Here's the drawing with two shaded views (mm, measured from the low corner). I have some questions. A direction names the side the tool comes from. Round coordinates to 2 decimals unless told otherwise and drop trailing zeros. Write each loop counter-clockwise with the first axis right and the second up, starting at its lowest first coordinate (ties: lowest second). Pieces come first, ordered by that corner, then holes. Notation, with made-up numbers: (13, 55.25) - (52, 55.25) arc R28 ccw to (52, 91.25) - close; hole circle Ø2 at (49.5, 79.5). An arc over 180 degrees is marked (long way). Return JSON: item names as keys, results as strings. Group by question number.
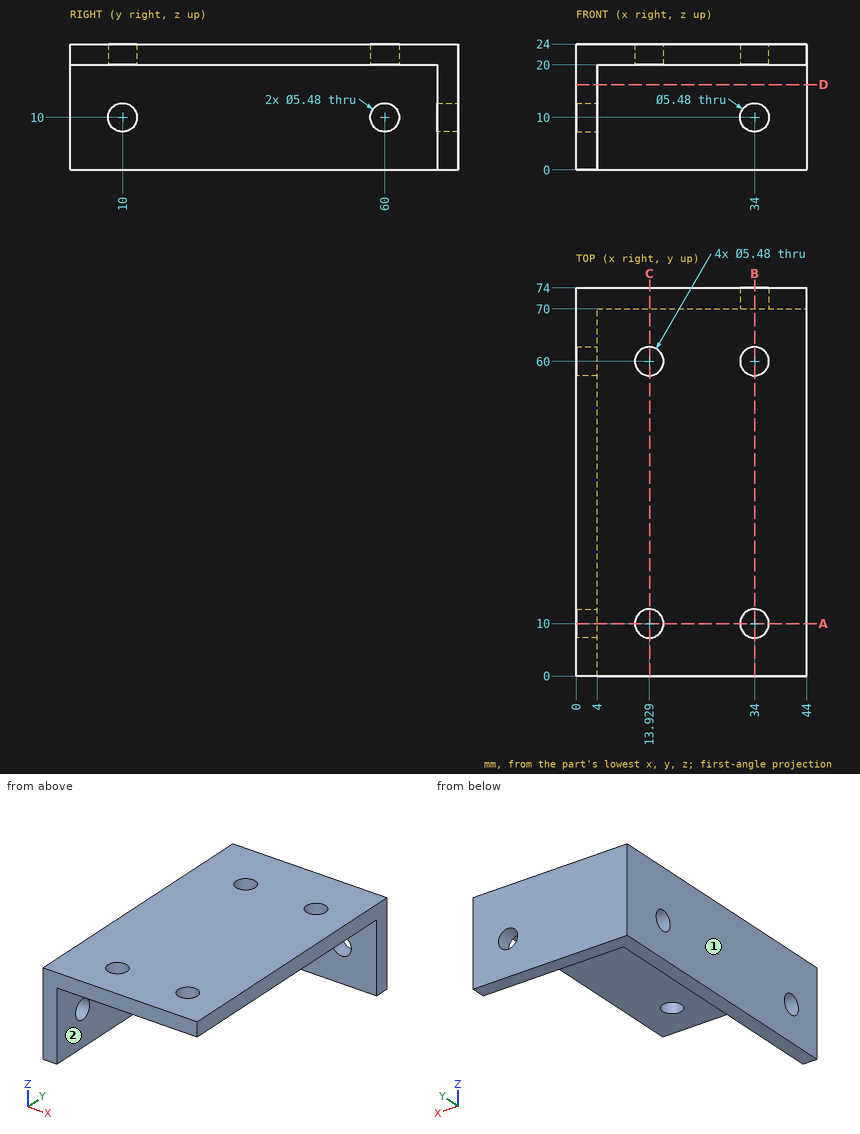
1) Imagine slicing it at A-A (y = 10). Please give me the cut outline in (x, z), plus the area to 3 significant figures.
2) Will these pins go through, and if not, where does the flat tip stop? pin 1 Ø6 at (x, y) = (6.5, 17.5) entering from -Z; pin 2 Ø2 at (y, z) = (34, 17) entering from +X; pin 3 Ø10 at (x, z) = (30.5, 14) entering from -Y; pin 4 Ø7 at (x, y) = (34, 10) entering from -Z.
3) For the marked faces 1 and 2, which set-ups out of +Z, -Z, +X, -X, +Y, -Y let a thin tool reach every point of the face, with its end or its side?
4) Imagine slicing it at B-B (x = 34). Please give me the cut outline in (y, z).
5) Imagine slicing it at D-D (z = 16.25). Please give me the cut outline in (x, y).
6) Imagine slicing it at C-C (x = 14). Please give me the cut outline in (y, z), plus the area to 3 significant figures.
7) I need wall thicknesses on line 1 along X through (y, z) = (10, 22.75); line 2 along Y through (x, z) = (34, 23.2); line 3 along Z through (x, y) = (2.25, 10). Which ranges of each line are inside material? Lowest first, please.
Results found:
{
 "1": {"outline": "(0, 0) - (4, 0) - (4, 7.26) - (0, 7.26) - close; (0, 12.74) - (4, 12.74) - (4, 20) - (11.19, 20) - (11.19, 24) - (0, 24) - close; (16.67, 20) - (31.26, 20) - (31.26, 24) - (16.67, 24) - close; (36.74, 20) - (44, 20) - (44, 24) - (36.74, 24) - close", "area": "190 mm²"},
 "2": {"pin 1": "stops at z = 0", "pin 2": "stops at x = 4", "pin 3": "stops at y = 70", "pin 4": "stops at z = 20"},
 "3": {"face 1": "+Z, -Z, -X, +Y, -Y", "face 2": "-Z, +X, -Y"},
 "4": {"outline": "(0, 20) - (7.26, 20) - (7.26, 24) - (0, 24) - close; (12.74, 20) - (57.26, 20) - (57.26, 24) - (12.74, 24) - close; (62.74, 20) - (70, 20) - (70, 12.74) - (74, 12.74) - (74, 24) - (62.74, 24) - close; (70, 0) - (74, 0) - (74, 7.26) - (70, 7.26) - close"},
 "5": {"outline": "(0, 0) - (4, 0) - (4, 70) - (44, 70) - (44, 74) - (0, 74) - close"},
 "6": {"outline": "(0, 20) - (7.26, 20) - (7.26, 24) - (0, 24) - close; (12.74, 20) - (57.26, 20) - (57.26, 24) - (12.74, 24) - close; (62.74, 20) - (70, 20) - (70, 0) - (74, 0) - (74, 24) - (62.74, 24) - close", "area": "332 mm²"},
 "7": {"line 1": "x = 0 to 11.19, 16.67 to 31.26, 36.74 to 44", "line 2": "y = 0 to 7.26, 12.74 to 57.26, 62.74 to 74", "line 3": "z = 0 to 7.26, 12.74 to 24"}
}
